The listing builds one solid part. Answer for the finished solid, in the listing's coordinates (mm). Face numbers are marked on the shaded views. A direction names the side the tool comes from. Coordinates: 2 decimals unless noted, no trailing zeros. Write each loop counter-clockwise with the first axis right and the second up, starting at its lowest first coordinate (ties: lowest second). Pieces come first, ordered by that corner, then holes.
(1) The part is cut by section B-B on y = 1.5. Determine the outline of the cut face in (x, z).
(2) The part is cut by section C-C on x = -14. Determine the outline of the cut face in (y, z).
(3) Which of the six approach directions +Z, -Z, +X, -X, +Y, -Y give full straight-line access (tool end or side, diameter ignored) to the marked faces 4, 5 and 6?
(4) Given P1, Ø2, axis at x = 5, z = 5, coming from the -Y side; P2, Ø2, axis at x = 13, y = 1.5, coming from the +Z side, each flat-ended and moving along its own axis, determine where each tip first touches the part or whether it passes through.
(5) For a pull along X with two mould halves and no side action, classify the marked faces 1, 2 and 3 as +X half, -X half, draft (parallel to the pull), parting line (faces both ways), or undercut.
(6) The part is cut by section D-D on y = 3.6. Determine the outline of the cut face in (x, z), plus the area to 3 significant figures.
(7) The part is cut by section A-A on z = -1.75. Determine the outline of the cut face in (x, y), plus the area to 3 significant figures.
(8) Straight lines are drawn through the part: line 1 (X direction, y = 1, z = -6.5); line 2 (Z direction, x = -14.5, y = 0.95); line 3 (Y direction, x = 9.5, z = 7.75). For each, find the intervals that lie inside material, in ascending order.
from build123d import *

# Parameters (mm, degrees)
CROQUIS1_W              = 34
CROQUIS1_H              = 17
SALIENTE_EXTRUIR1_DEPTH = 4
CROQUIS2_W              = 16
CROQUIS2_H              = 9
CORTAR_EXTRUIR1_DEPTH   = 5
CROQUIS3_W              = 34
CROQUIS3_H              = 2.7
CORTAR_EXTRUIR2_DEPTH   = 8
CORTAR_EXTRUIR3_DEPTH   = 3
REDONDEO3_R             = 1
REDONDEO4_R             = 1


with BuildPart() as part:
    # Croquis1 → Saliente-Extruir1 (new body)
    with BuildSketch(Plane(origin=(0, 0, 0), x_dir=(1, 0, 0), z_dir=(0, 1, 0))):
        Rectangle(CROQUIS1_W, CROQUIS1_H)
    extrude(amount=SALIENTE_EXTRUIR1_DEPTH)

    # Croquis2 → Cortar-Extruir1 (cut)
    with BuildSketch(Plane(origin=(0, 4, 0), x_dir=(1, 0, 0), z_dir=(0, 1, 0))):
        with Locations((0, 4)):
            Rectangle(CROQUIS2_W, CROQUIS2_H)
    extrude(amount=-CORTAR_EXTRUIR1_DEPTH, mode=Mode.SUBTRACT)

    # Croquis3 → Cortar-Extruir2 (cut)
    with BuildSketch(Plane.XY.offset(8.5)):
        with Locations((0, 1.35)):
            Rectangle(CROQUIS3_W, CROQUIS3_H)
    extrude(amount=-CORTAR_EXTRUIR2_DEPTH, mode=Mode.SUBTRACT)

    # Croquis4 → Cortar-Extruir3 (cut)
    with BuildSketch(Plane(origin=(0, 4, 0), x_dir=(1, 0, 0), z_dir=(0, 1, 0))):
        Polygon((-17, -0.5), (-13, -8.5), (-17, -8.5), align=None)
        Polygon((13, -8.5), (17, -8.5), (17, -0.5), align=None)
    extrude(amount=-CORTAR_EXTRUIR3_DEPTH, mode=Mode.SUBTRACT)

    # Redondeo3
    redondeo3_edges = [part.edges().sort_by_distance(p)[0] for p in [
        (-13, 3.35, 8.5),
    ]]
    fillet(redondeo3_edges, radius=REDONDEO3_R)

    # Redondeo4
    redondeo4_edges = [part.edges().sort_by_distance(p)[0] for p in [
        (13, 3.35, 8.5),
    ]]
    fillet(redondeo4_edges, radius=REDONDEO4_R)


solid = part.part
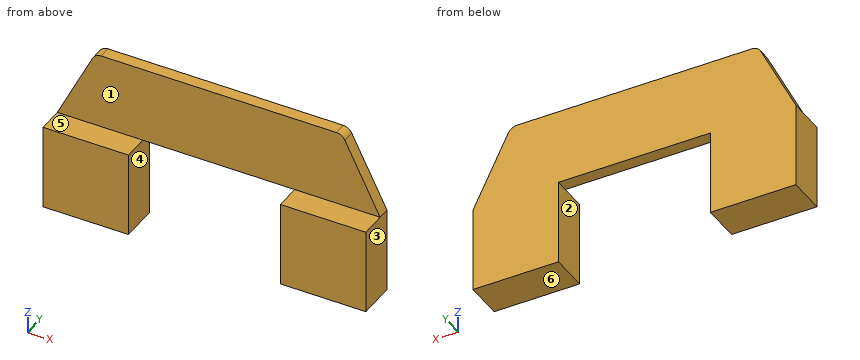
Model answer:
1. outline: (-17, -8.5) - (-8, -8.5) - (-8, 0.5) - (-17, 0.5) - close; (8, -8.5) - (17, -8.5) - (17, 0.5) - (8, 0.5) - close
2. outline: (0, -8.5) - (4, -8.5) - (4, 6.5) - (2.7, 6.5) - (2.7, 0.5) - (0, 0.5) - close
3. face 4: -Z, +Y, -Y
3. face 5: +Z, +X, -X, -Y
3. face 6: -Z, +X, -X, +Y, -Y
4. P1: stops at y = 2.7
4. P2: stops at z = 0.5
5. face 1: draft
5. face 2: undercut
5. face 3: +X half
6. outline: (-17, -8.5) - (-8, -8.5) - (-8, 0.5) - (8, 0.5) - (8, -8.5) - (17, -8.5) - (17, 0.5) - (13.28, 7.95) arc R1 ccw to (12.38, 8.5) - (-12.38, 8.5) arc R1 ccw to (-13.28, 7.95) - (-17, 0.5) - close
6. area: 402 mm2
7. outline: (-17, 0) - (-8, 0) - (-8, 4) - (-17, 4) - close; (8, 0) - (17, 0) - (17, 4) - (8, 4) - close
7. area: 72.0 mm2
8. line 1: x = -17 to -8, 8 to 17
8. line 2: z = -8.5 to 0.5
8. line 3: y = 2.7 to 4
